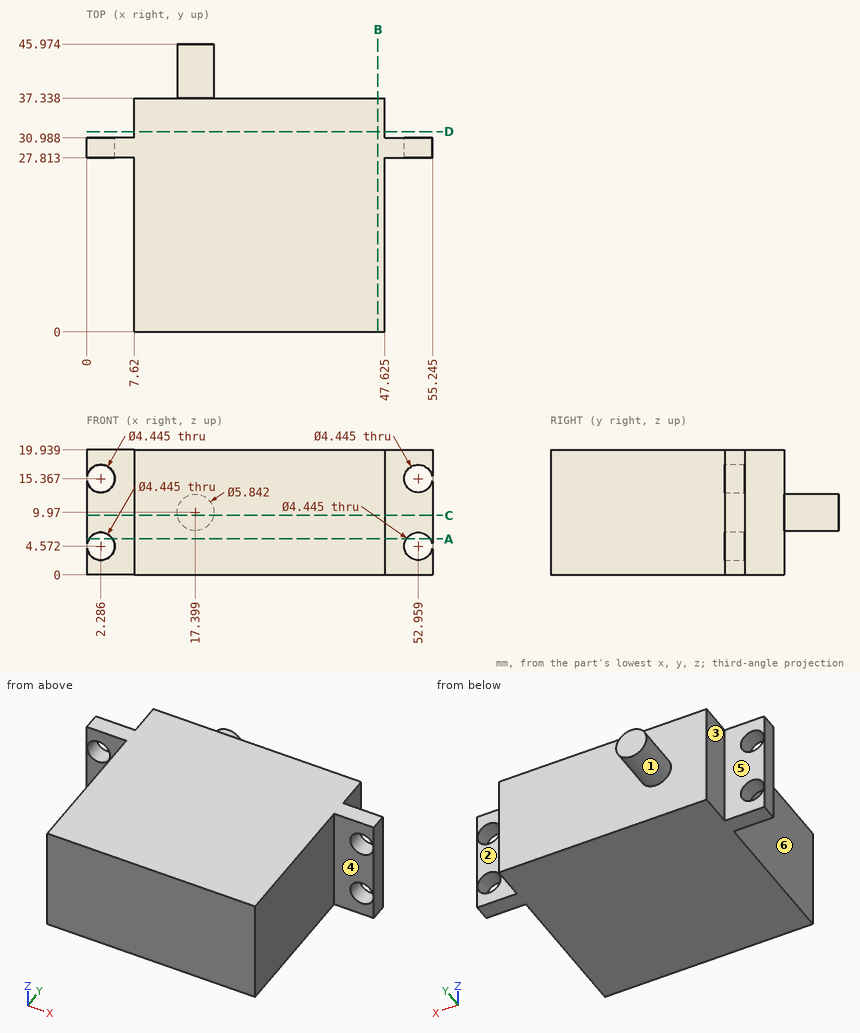
Check sheet for the drawn part. Datum: minimum x, y, z corner. Units: mm. A direction names the side the tool comes from. Give positions to 0.01 mm unless a question says otherwise; leave off trailing zeros. Order: outer loops, then holes, each group sorted by start corner. A loop starts at its lowest first (then second) coordinate and runs counter-clockwise, first axis right, second up. Notation, with made-up numbers: (-28.75, 32.25) - (-6.75, 32.25) arc R17 cw to (-6.75, 50.25) - close; hole circle Ø7 at (-24.75, 25.25). An arc over 180 degrees is marked (long way). Answer as a JSON object with one key per item and string values.
(1) Draft check along X on the marked faces 1, 2 and 3. Enter one of: released by +X, released by -X, zero draft, split by the parting line, or undercut.
Report:
{"face 1": "split by the parting line", "face 2": "zero draft", "face 3": "released by -X"}
(2) Material ranges on line 1 (X direction, y = 7, z = 15.75) (1 decimal); line 2 (Y direction, x = 40.5, z = 9.25); line 3 (Y direction, x = 52, z = 19), recorded low to high.
Report:
{"line 1": "7.6 to 47.6", "line 2": "0 to 37.34", "line 3": "27.81 to 30.99"}
(3) Depth check by flat-ended pin: pin 1 Ø4 at (x, z) = (52.959, 4.572) entering from -Y; pin 2 Ø6 at (y, z) = (14.5, 8) entering from +X (1 decimal); pin 3 Ø5 at (x, z) = (2.286, 15.367) entering from -Y; pin 4 Ø6 at (x, z) = (2.286, 4.572) entering from +Y. Enter the tip coordinate at first touch or a pass-through.
Report:
{"pin 1": "through", "pin 2": "x = 47.6", "pin 3": "y = 27.81", "pin 4": "y = 30.99"}
(4) Tool access check on the marked faces 4, 5 and 6. Record the directions out of +Z, -Z, +X, -X, +Y, -Y that give a thin tool (end or side, any length) a straight path to the whole face; none if there is none.
Report:
{"face 4": "+Z, -Z, +X, -Y", "face 5": "+Z, -Z, -X, +Y", "face 6": "+Z, -Z, -X, -Y"}
(5) Cross-section at D-D (y = 32). Record the cut outline in (x, z) (1 decimal), then the cut area to 3 significant figures.
Report:
{"outline": "(7.6, 0) - (47.6, 0) - (47.6, 19.9) - (7.6, 19.9) - close", "area": "798 mm^2"}
(6) Cross-section at A-A (z = 5.75). Record the cut outline in (x, y) (1 decimal), then the cut area to 3 significant figures.
Report:
{"outline": "(0, 27.8) - (0.4, 27.8) - (0.4, 31) - (0, 31) - close; (4.2, 27.8) - (7.6, 27.8) - (7.6, 0) - (47.6, 0) - (47.6, 27.8) - (51.1, 27.8) - (51.1, 31) - (47.6, 31) - (47.6, 37.3) - (7.6, 37.3) - (7.6, 31) - (4.2, 31) - close; (54.8, 27.8) - (55.2, 27.8) - (55.2, 31) - (54.8, 31) - close", "area": "1,520 mm^2"}
(7) Cross-section at C-C (z = 9.5). Record the cut outline in (x, y) (1 decimal), then the cut area to 3 significant figures.
Report:
{"outline": "(0, 27.8) - (7.6, 27.8) - (7.6, 0) - (47.6, 0) - (47.6, 27.8) - (55.2, 27.8) - (55.2, 31) - (47.6, 31) - (47.6, 37.3) - (20.3, 37.3) - (20.3, 46) - (14.5, 46) - (14.5, 37.3) - (7.6, 37.3) - (7.6, 31) - (0, 31) - close", "area": "1,590 mm^2"}
(8) Cross-section at B-B (x = 46.5). Record the cut outline in (y, z).
Report:
{"outline": "(0, 0) - (37.34, 0) - (37.34, 19.94) - (0, 19.94) - close"}
